```python
from build123d import *

# Parameters (mm, degrees)
BOSS_EXTRUDE1_DEPTH = 5
SKETCH2_R           = 1.5
CUT_EXTRUDE1_DEPTH  = 7
SKETCH3_R           = 1.5
CUT_EXTRUDE2_DEPTH  = 7
SKETCH4_R           = 1.5
CUT_EXTRUDE3_DEPTH  = 7


with BuildPart() as part:
    # Sketch1 → Boss-Extrude1 (new body)
    with BuildSketch(Plane(origin=(0, 0, 0), x_dir=(1, 0, 0), z_dir=(0, 1, 0))):
        Polygon((0, 0), (-20, 0), (0, 20), align=None)
    extrude(amount=BOSS_EXTRUDE1_DEPTH)

    # Sketch2 → Cut-Extrude1 (cut)
    with BuildSketch(Plane.XY):
        with Locations((-10, 2.5)):
            Circle(SKETCH2_R)
    extrude(amount=-CUT_EXTRUDE1_DEPTH, mode=Mode.SUBTRACT)

    # Sketch3 → Cut-Extrude2 (cut)
    with BuildSketch(Plane(origin=(-10, 0, -10), x_dir=(-0.7071067811865511, 0, 0.7071067811865439), z_dir=(-0.7071067811865439, 0, -0.7071067811865511))):
        with Locations((-3.357864376, 2.5)):
            Circle(SKETCH3_R)
    extrude(amount=-CUT_EXTRUDE2_DEPTH, mode=Mode.SUBTRACT)

    # Sketch4 → Cut-Extrude3 (cut)
    with BuildSketch(Plane(origin=(0, 5, 0), x_dir=(1, 0, 0), z_dir=(0, 1, 0))):
        with Locations(Location((-4, 3, 0), (0, 0, 270))):
            Circle(SKETCH4_R)
    extrude(amount=-CUT_EXTRUDE3_DEPTH, mode=Mode.SUBTRACT)


solid = part.part
```
Could you check a few things on this model? Use its own coordinates, in mm. A direction names the side the tool comes from. Coordinates: 2 decimals unless noted, no trailing zeros. Order: outer loops, then holes, each group sorted by start corner. A loop starts at its lowest first (then second) coordinate and runs counter-clockwise, first axis right, second up. Notation, with made-up numbers: M 60,-35 L 75,-35 A29 ccw 75,-3 Z; hole C -26,63 d5. An arc over 180 degrees is marked long. Use one line per item in the form item = value. Start each with the question number.
1. We'd pull the mould along X, two halves only. Please class faces 4 (the flat face through (0, 2, -10)), 5 (the flat face through (-10, 2, -10)), 6 (the flat face through (-10, 3, -7)): +X half, -X half, draft (parallel to the pull), parting line (faces both ways), or undercut.
2. Please list where these lines run through material, in increasing order: line 1 (Y direction, x = -10, z = -2.75); line 2 (X direction, y = 3.3, z = -3.5); line 3 (X direction, y = 1.3, z = -3).
3. Suppose I cut it at B-B on x = -10. Write out the boundary of the cut face in (y, z).
4. On a 3-axis mill with a long thin cutter (end or side, diameter ignored), from which of +Z, -Z, +X, -X, +Y, -Y can I reach the whole of each face in a straight line? I mean faces 1 (the flat face through (-9.9, 0.8, 0)), 2 (the cylindrical face through (-11.2, 1.6, -3.5)), 3 (the flat face through (-2.7, 2.5, -7.4)). Say none if no direction works.
5. Suppose I cut it at C-C on y = 2.5. Write out the boundary of the cut face in (x, z).
6. For pin 1 (1.5 mm diameter, centred on y = 2, z = -2.5, fed in from -X); pin 2 (2 mm diameter, centred on x = -2.5, y = 1.5, fed in from -Z), each with a flat end and sliding along its axis, tell me the tip position at first contact or that it passes through.
7. Suppose I cut it at A-A on z = -3. Write out the boundary of the cut face in (x, y).
8. Suppose I cut it at D-D on x = -4. Count the separate pieces of the cut face and the enclosed holes in it, then the cut area to 3 significant figures.
Geometry says:
q1.face_4 = +X half
q1.face_5 = -X half
q1.face_6 = undercut
q2.line_1 = 0 to 1, 4 to 5
q2.line_2 = -16.5 to -11.27, -8.73 to -5.41, -2.59 to 0
q2.line_3 = -17 to -10.9, -9.1 to -5.5, -2.5 to 0
q3.outline = M 0,-10 L 5,-10 L 5,0 L 4,0 L 4,-7 L 1,-7 L 1,0 L 0,0 Z
q4.face_1 = +Z, +X, -X, +Y, -Y
q4.face_2 = +Z
q4.face_3 = none
q5.outline = M -20,0 L -8.69,-11.31 L -3.74,-6.36 L -1.62,-8.49 L -6.56,-13.44 L 0,-20 L 0,0 L -8.5,0 L -8.5,-7 L -11.5,-7 L -11.5,0 Z; hole C -4,-3 d3
q6.pin_1 = -18.25
q6.pin_2 = -18.5
q7.outline = M -17,0 L -5.5,0 L -5.5,5 L -17,5 Z; M -2.5,0 L 0,0 L 0,5 L -2.5,5 Z; hole C -10,2.5 d3
q8.separate_pieces = 2
q8.enclosed_holes = 1
q8.area = 55.0 mm^2
